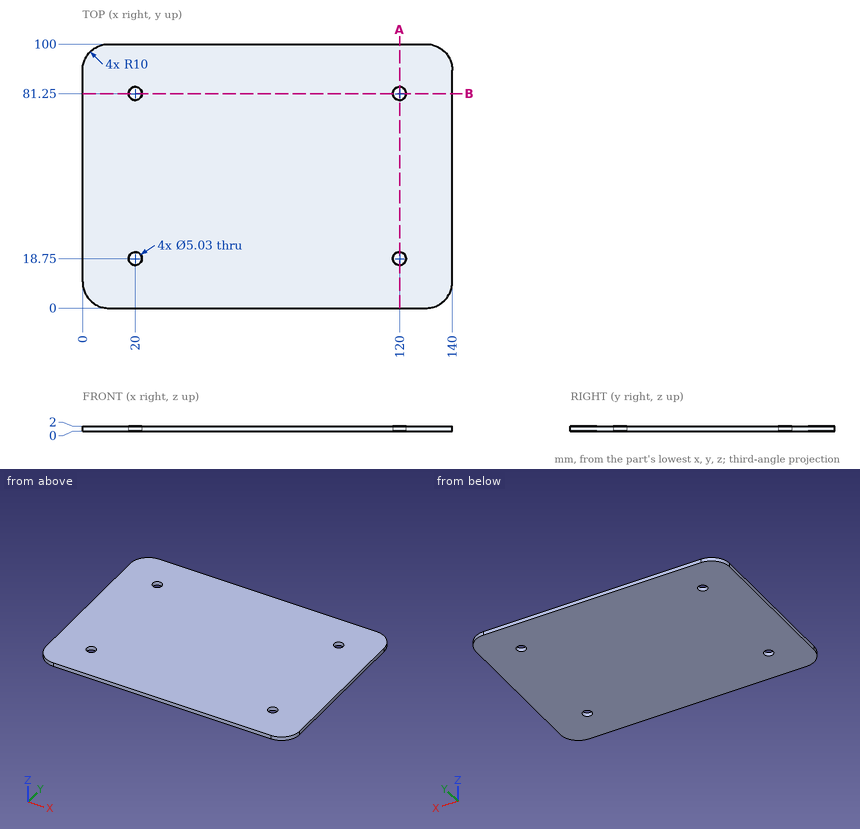
Can you work these out from the drawing? Everything is in mm from the part's minimum corner. Coordinates: 2 decimals unless noted, no trailing zeros. Loops run counter-clockwise (first coordinate to the right, second up) from the corner with the lowest first, then second, coordinate; pieces in that order, holes last.
1) Imagine slicing it at A-A on x = 120. List the corners of the cut face in (y, z) for me (3 decimals), plus the area to 3 significant figures.
2) Imagine slicing it at B-B on y = 81.25. List the corners of the cut face in (x, z) for me (3 decimals).
3) I need wall thicknesses on probe 1 along X at (y, z) = (81.25, 1.6) (3 decimals); probe 2 along Y at (x, z) = (120, 0.8) (3 decimals); probe 3 along Y at (x, z) = (21, 0.4). Which ranges of each line are inside material? Lowest first, please.
Completed:
1. outline: (0, 0) - (16.235, 0) - (16.235, 2) - (0, 2) - close; (21.265, 0) - (78.735, 0) - (78.735, 2) - (21.265, 2) - close; (83.765, 0) - (100, 0) - (100, 2) - (83.765, 2) - close
1. area: 180 mm2
2. outline: (0, 0) - (17.485, 0) - (17.485, 2) - (0, 2) - close; (22.515, 0) - (117.485, 0) - (117.485, 2) - (22.515, 2) - close; (122.515, 0) - (140, 0) - (140, 2) - (122.515, 2) - close
3. probe 1: x = 0 to 17.485, 22.515 to 117.485, 122.515 to 140
3. probe 2: y = 0 to 16.235, 21.265 to 78.735, 83.765 to 100
3. probe 3: y = 0 to 16.44, 21.06 to 78.94, 83.56 to 100
